For this review, take the finished solid that the model builds, in its own axes (mm). Coordinates: 2 decimals unless noted, no trailing zeros. Order: outer loops, then holes, each group sorted by start corner. A loop starts at its lowest first (then second) coordinate and runs counter-clockwise, first axis right, second up.
from build123d import *

# Parameters (mm, degrees)
F0_W     = 2
F0_H     = 4.9
F0_W_2   = 4.9
F0_H_2   = 3
F2_DEPTH = 2
F3_DEPTH = 12.5


with BuildPart() as f2:
    # F0 (on Top) → F2 (new body)
    with BuildSketch(Plane.XY):
        with Locations((44, -20)):
            Rectangle(F0_W, F0_H)
        with Locations((-7.5, -54)):
            Rectangle(F0_W_2, F0_H_2)
        with Locations((44, 30)):
            Rectangle(F0_W, F0_H)
        with Locations((17.5, -54)):
            Rectangle(F0_W_2, F0_H_2)
        with Locations((44, 20)):
            Rectangle(F0_W, F0_H)
        with Locations((-44, 30)):
            Rectangle(F0_W, F0_H)
        with Locations((-44, -30)):
            Rectangle(F0_W, F0_H)
        with Locations((44, 10)):
            Rectangle(F0_W, F0_H)
        with Locations((-44, 40)):
            Rectangle(F0_W, F0_H)
        with Locations((-44, -40)):
            Rectangle(F0_W, F0_H)
        with Locations((44, -10)):
            Rectangle(F0_W, F0_H)
        with Locations((-44, 20)):
            Rectangle(F0_W, F0_H)
        with Locations((-44, -20)):
            Rectangle(F0_W, F0_H)
        with Locations((44, 40)):
            Rectangle(F0_W, F0_H)
        with Locations((-44, 10)):
            Rectangle(F0_W, F0_H)
        with Locations((-44, -10)):
            Rectangle(F0_W, F0_H)
        with Locations((-27.5, -54)):
            Rectangle(F0_W_2, F0_H_2)
        with Locations((7.5, -54)):
            Rectangle(F0_W_2, F0_H_2)
        with Locations((-17.5, -54)):
            Rectangle(F0_W_2, F0_H_2)
        with Locations((-37.5, -54)):
            Rectangle(F0_W_2, F0_H_2)
        Polygon((43, 52.5), (-43, 52.5), (-43, 42.45), (-43, 37.55), (-43, 32.45), (-43, 27.55), (-43, 22.45), (-43, 17.55), (-43, 12.45), (-43, 7.55), (-43, -7.55), (-43, -12.45), (-43, -17.55), (-43, -22.45), (-43, -27.55), (-43, -32.45), (-43, -37.55), (-43, -42.45), (-43, -52.5), (-39.95, -52.5), (-35.05, -52.5), (-29.95, -52.5), (-25.05, -52.5), (-19.95, -52.5), (-15.05, -52.5), (-9.95, -52.5), (-5.05, -52.5), (5.05, -52.5), (9.95, -52.5), (15.05, -52.5), (19.95, -52.5), (25.05, -52.5), (29.95, -52.5), (35.05, -52.5), (39.95, -52.5), (43, -52.5), (43, -42.45), (43, -37.55), (43, -32.45), (43, -27.55), (43, -22.45), (43, -17.55), (43, -12.45), (43, -7.55), (43, 7.55), (43, 12.45), (43, 17.55), (43, 22.45), (43, 27.55), (43, 32.45), (43, 37.55), (43, 42.45), align=None)
        with Locations((27.5, -54)):
            Rectangle(F0_W_2, F0_H_2)
        with Locations((44, -30)):
            Rectangle(F0_W, F0_H)
        with Locations((37.5, -54)):
            Rectangle(F0_W_2, F0_H_2)
        with Locations((44, -40)):
            Rectangle(F0_W, F0_H)
    extrude(amount=F2_DEPTH)

    # F1 (on face) → F3 (cut, symmetric)
    with BuildSketch(Plane.XY):
        Polygon((-23.174025, -19.499996), (-33.56633, -13.5), (-33.56633, -37.5), (-23.174025, -31.499996), align=None)
        Polygon((-33.56633, 1.964102), (-23.174025, 7.964102), (-23.174025, 19.964102), (-33.56633, 25.964102), align=None)
        Polygon((-10.78172, 1.964102), (-0.389415, 7.964102), (-0.389415, 19.964102), (-10.78172, 25.964102), (-21.174025, 19.964102), (-21.174025, 7.964102), align=None)
        Polygon((12.00289, 1.964102), (22.395195, 7.964102), (22.395195, 19.964102), (12.00289, 25.964102), (1.610585, 19.964102), (1.610585, 7.964102), align=None)
        Polygon((24.395195, 7.964102), (34.787499, 1.964102), (34.787499, 25.964102), (24.395195, 19.964102), align=None)
        Polygon((34.787499, -37.5), (34.787499, -13.5), (24.395195, -19.5), (24.395195, -31.5), align=None)
        Polygon((-22.174025, -17.767949), (-11.78172, -11.767949), (-11.78172, 0.232051), (-22.174025, 6.232051), (-32.56633, 0.232051), (-32.56633, -11.767949), align=None)
        Polygon((0.610585, -17.767949), (11.00289, -11.767949), (11.00289, 0.232051), (0.610585, 6.232051), (-9.78172, 0.232051), (-9.78172, -11.767949), align=None)
        Polygon((23.395195, -17.767949), (33.787499, -11.767949), (33.787499, 0.232051), (23.395195, 6.232051), (13.00289, 0.232051), (13.00289, -11.767949), align=None)
        Polygon((-10.78172, -37.5), (-0.389415, -31.5), (-0.389415, -19.5), (-10.78172, -13.5), (-21.174025, -19.5), (-21.174025, -31.5), align=None)
        Polygon((12.00289, -37.5), (22.395195, -31.5), (22.395195, -19.5), (12.00289, -13.5), (1.610585, -19.5), (1.610585, -31.5), align=None)
    extrude(amount=F3_DEPTH, both=True, mode=Mode.SUBTRACT)


solid = f2.part
1. The part is to be moulded in two halves that separate along Y. For faces 1 (the face through (-27.297, 3.274, 0.986)), 2 (the face through (-11, -1, 2)), say which applies: +Y half, -Y half, draft (parallel to the pull), parting line (faces both ways), or undercut.
Answer below:
face 1: undercut
face 2: draft
2. Take a section at D-D, the plane y = -48. Give the boundary of the cut face in (x, z), plus the area to 3 significant figures.
Answer below:
outline: (-43, 0) - (43, 0) - (43, 2) - (-43, 2) - close
area: 172 mm2
3. Clearance check with flat-ended pins moving along their axes: pin 1 Ø0.6 at (y, z) = (-34.5, 1.5) entering from -X; pin 2 Ø0.6 at (x, z) = (44, 1) entering from +Y; pin 3 Ø0.6 at (x, z) = (-41, 1.5) entering from -Y. State where each tip first meets the part, or that it passes through.
Answer below:
pin 1: stops at x = -43
pin 2: stops at y = 42.45
pin 3: stops at y = -52.5
4. Take a section at C-C, the plane z = 1. Give the number of separate pieces and of enclosed holes in the cut face, plus the area to 3 significant figures.
Answer below:
separate pieces: 1
enclosed holes: 11
area: 5,940 mm2
5. Take a section at B-B, the plane x = -28. Give the boundary of the cut face in (y, z).
Answer below:
outline: (-55.5, 0) - (-34.29, 0) - (-34.29, 2) - (-55.5, 2) - close; (-16.71, 0) - (-14.4, 0) - (-14.4, 2) - (-16.71, 2) - close; (2.87, 0) - (5.18, 0) - (5.18, 2) - (2.87, 2) - close; (22.75, 0) - (52.5, 0) - (52.5, 2) - (22.75, 2) - close
6. To check wall thickness, follow L1, parallel to X at y = -11.5, z = 1.25; L2, parallel to X at y = 13.5, z = 0.8; L3, parallel to X at y = 19.5, z = 1.85. State the ranges of each line that lie inside material, in increasing order.
Answer below:
L1: x = -45 to -32.57, -11.78 to -9.78, 11 to 13, 33.79 to 45
L2: x = -43 to -33.57, -23.17 to -21.17, -0.39 to 1.61, 22.4 to 24.4, 34.79 to 43
L3: x = -45 to -33.57, -23.17 to -21.17, -0.39 to 1.61, 22.4 to 24.4, 34.79 to 45
7. Take a section at A-A, the plane y = 9.5. Give the boundary of the cut face in (x, z).
Answer below:
outline: (-45, 0) - (-33.57, 0) - (-33.57, 2) - (-45, 2) - close; (-23.17, 0) - (-21.17, 0) - (-21.17, 2) - (-23.17, 2) - close; (-0.39, 0) - (1.61, 0) - (1.61, 2) - (-0.39, 2) - close; (22.4, 0) - (24.4, 0) - (24.4, 2) - (22.4, 2) - close; (34.79, 0) - (45, 0) - (45, 2) - (34.79, 2) - close
